```python
from build123d import *

# Parameters (mm, degrees)
BOSS_EXTRUDE1_DEPTH    = 25.4
SKETCH2_R              = 2.159
SKETCH2_W              = 12.7
SKETCH2_H              = 1.5875
SKETCH2_W_2            = 1.5875
SKETCH2_H_2            = 12.7
CUT_EXTRUDE1_DEPTH     = 25.4
SKETCH3_W              = 12.7
SKETCH3_H              = 1.5875
SKETCH3_H_2            = 1.5748
CUT_EXTRUDE2_DEPTH     = 12.7
SKETCH4_W              = 1.5875
SKETCH4_H              = 12.7
CUT_EXTRUDE3_DEPTH     = 12.7
F_3DSKETCH1_R          = 19.05
F_3DSKETCH1_R_2        = 11.1125
BOSS_EXTRUDE2_DEPTH    = 11.482870812
CUT_EXTRUDE4_START     = 44.901280605
CUT_EXTRUDE4_OUTLINE_R = 11.1125
CUT_EXTRUDE4_DEPTH     = 11.482870812


# Read off the part's stored shape, not the designer's step: Cut-Extrude4
with BuildPart() as part:
    # Sketch1 → Boss-Extrude1 (new body)
    with BuildSketch(Plane.XY):
        Polygon((88.9, 0), (63.5, 0), (0, -63.5), (0, -88.9), (12.7, -88.9), (12.7, -67.039231637), (67.039231637, -12.7), (88.9, -12.7), align=None)
    extrude(amount=BOSS_EXTRUDE1_DEPTH)

    # Sketch2 → Cut-Extrude1 (cut)
    with BuildSketch(Plane.XY.offset(25.4)):
        with Locations((82.55, -6.3627)):
            Circle(SKETCH2_R)
        with Locations((6.3627, -82.55)):
            Circle(SKETCH2_R)
        with Locations((82.55, -0.79375)):
            Rectangle(SKETCH2_W, SKETCH2_H)
        with Locations((0.79375, -82.55)):
            Rectangle(SKETCH2_W_2, SKETCH2_H_2)
    extrude(amount=-CUT_EXTRUDE1_DEPTH, mode=Mode.SUBTRACT)

    # Sketch3 → Cut-Extrude2 (cut)
    with BuildSketch(Plane.XZ.offset(88.9)):
        with Locations((6.35, 24.60625)):
            Rectangle(SKETCH3_W, SKETCH3_H)
        with Locations((6.35, 0.7874)):
            Rectangle(SKETCH3_W, SKETCH3_H_2)
    extrude(amount=-CUT_EXTRUDE2_DEPTH, mode=Mode.SUBTRACT)

    # Sketch4 → Cut-Extrude3 (cut)
    with BuildSketch(Plane(origin=(88.9, 0, 0), x_dir=(0, 0, -1), z_dir=(1, 0, 0))):
        with Locations((-0.79375, -6.35)):
            Rectangle(SKETCH4_W, SKETCH4_H)
        with Locations((-24.60625, -6.35)):
            Rectangle(SKETCH4_W, SKETCH4_H)
    extrude(amount=-CUT_EXTRUDE3_DEPTH, mode=Mode.SUBTRACT)

    # 3DSketch1 → Boss-Extrude2 (add)
    with BuildSketch(Plane(origin=(67.039231637, -12.7, 0), x_dir=(-0.6713837490692134, -0.6713837490692195, 0.3138275369873187), z_dir=(0.7071067811865508, -0.7071067811865444, 0))):
        with Locations((40.468086778, 0)):
            Circle(F_3DSKETCH1_R)
        with Locations((40.468086778, 0)):
            Circle(F_3DSKETCH1_R_2, mode=Mode.SUBTRACT)
    extrude(amount=-BOSS_EXTRUDE2_DEPTH)

    # Cut-Extrude4 outline → Cut-Extrude4 (cut)
    with BuildSketch(Plane(origin=(0, 0, 0), x_dir=(0.7071067811865438, 0.7071067811865512, 0), z_dir=(0.7071067811865511, -0.7071067811865441, 0)).offset(CUT_EXTRUDE4_START)):
        with Locations((0, 12.7)):
            Circle(CUT_EXTRUDE4_OUTLINE_R)
    extrude(amount=CUT_EXTRUDE4_DEPTH, mode=Mode.SUBTRACT)


solid = part.part
```
Model file for the job. Use its own axes, mm. A direction names the side the tool comes from. Coordinates: 2 decimals unless noted, no trailing zeros. Loops run counter-clockwise (first coordinate to the right, second up) from the corner with the lowest first, then second, coordinate; pieces in that order, holes last. Notation, with made-up numbers: (33, 71) - (59, 71) arc R24 ccw to (59, 107) - close; hole circle Ø10 at (85.5, 34). An arc over 180 degrees is marked (long way). Answer as a JSON object with one key per item and string values. Group by question number.
(1) Tool access for faces 5 (the face through (84.1, -8.5, 23.812)), 6 (the face through (12.7, -78, 13)), 7 (the face through (8.3, -84.1, 23.812)), 8 (the face through (1.588, -83, 13)): list every direction of +Z, -Z, +X, -X, +Y, -Y with a clear straight run to the whole face (end or side of a thin tool).
(2) Cut at D-D (z = 11). Give the cut face in (x, y), then the cut area to 3 significant figures.
(3) Two-plate mould, pull along X, no slides. Class faces 1 (the face through (82, -1.588, 13)), 2 (the face through (35.71, -36.03, -6.35)), 3 (the face through (34.05, -37.456, 1.852)), 4 (the face through (45.53, -34.21, 20.9)): released by +X, released by -X, zero draft, split by the parting line, or undercut.
(4) Cut at B-B (z = 22.5). Give the cut face in (x, y).
(5) Probe line 1 along Y through (x, z) = (82.55, 13); line 2 along Y through (x, z) = (84.5, 13); line 3 along Z through (x, y) = (59.5, -13.5). List the from-to ranges inside material, lowest first.
(6) Flat gauge pins, fed straight in: pin 1 (10 mm diameter, centred on x = 17, y = -74.5, fed in from -Z); pin 2 (5.5 mm diameter, centred on x = 82, y = -9.5, fed in from -Z); pin 3 (4 mm diameter, centred on y = -54.5, z = 3.5, fed in from -X). Where does each tip first touch, or does it go through?
(7) Cut at C-C (x = 82.55). Give the cut face in (y, z), then the cut area to 3 significant figures.
(8) Cut at A-A (y = -82.55). Give the cut face in (x, z).
Geometry says:
{
 "1": {"face 5": "+Z, +X, +Y, -Y", "face 6": "+Z, -Z, +X, -Y", "face 7": "+Z, +X, -X, -Y", "face 8": "+Z, -Z, -X, -Y"},
 "2": {"outline": "(0, -76.2) - (1.59, -76.2) - (1.59, -88.9) - (12.7, -88.9) - (12.7, -67.04) - (32.1, -47.63) - (23.98, -39.52) - (0, -63.5) - close; (39.52, -23.98) - (47.63, -32.1) - (67.04, -12.7) - (88.9, -12.7) - (88.9, -1.59) - (76.2, -1.59) - (76.2, 0) - (63.5, 0) - close; hole circle Ø4.32 at (6.36, -82.55); hole circle Ø4.32 at (82.55, -6.36)", "area": "1,240 mm^2"},
 "3": {"face 1": "zero draft", "face 2": "split by the parting line", "face 3": "undercut", "face 4": "released by +X"},
 "4": {"outline": "(0, -76.2) - (1.59, -76.2) - (1.59, -88.9) - (12.7, -88.9) - (12.7, -67.04) - (36.17, -43.57) - (28.05, -35.45) - (0, -63.5) - close; (35.45, -28.05) - (43.57, -36.17) - (67.04, -12.7) - (88.9, -12.7) - (88.9, -1.59) - (76.2, -1.59) - (76.2, 0) - (63.5, 0) - close; hole circle Ø4.32 at (6.36, -82.55); hole circle Ø4.32 at (82.55, -6.36)"},
 "5": {"line 1": "y = -12.7 to -8.52, -4.2 to -1.59", "line 2": "y = -12.7 to -7.29, -5.44 to -1.59", "line 3": "z = 0 to 25.4"},
 "6": {"pin 1": "stops at z = 0", "pin 2": "stops at z = 1.59", "pin 3": "stops at x = 7"},
 "7": {"outline": "(-12.7, 1.59) - (-8.52, 1.59) - (-8.52, 23.81) - (-12.7, 23.81) - close; (-4.2, 1.59) - (-1.59, 1.59) - (-1.59, 23.81) - (-4.2, 23.81) - close", "area": "151 mm^2"},
 "8": {"outline": "(1.59, 1.57) - (4.2, 1.57) - (4.2, 23.81) - (1.59, 23.81) - close; (8.52, 1.57) - (12.7, 1.57) - (12.7, 23.81) - (8.52, 23.81) - close"}
}
